from build123d import *

# Parameters (mm, degrees)
SKETCH1_W               = 1019.556
SKETCH1_H               = 756.92
BOSS_EXTRUDE1_DEPTH     = 800
CUT_EXTRUDE1_DEPTH      = 1351.083852483
CUT_EXTRUDE2_DEPTH      = 1022.325404014
CUT_EXTRUDE2_DEPTH_BACK = 1022.325404014


with BuildPart() as part:
    # Sketch1 → Boss-Extrude1 (new body)
    with BuildSketch(Plane.XY):
        Rectangle(SKETCH1_W, SKETCH1_H)
    extrude(amount=BOSS_EXTRUDE1_DEPTH)

    # Sketch2 → Cut-Extrude1 (cut, through all)
    with BuildSketch(Plane(origin=(509.778, 0, 0), x_dir=(0, 0, -1), z_dir=(1, 0, 0))):
        Polygon((2016.625671317, 1289.001404615), (0, 378.46), (-838.195987242, 0), (0, -378.46), (2016.625671317, -1289.001404615), (-2408.694542061, -1289.001404615), (-2408.694542061, 1289.001404615), align=None)
    extrude(amount=-CUT_EXTRUDE1_DEPTH, mode=Mode.SUBTRACT)

    # Sketch4 → Cut-Extrude2 (cut, two sides: drawn at the far end of the back side and taken through both)
    with BuildSketch(Plane(origin=(0, 0, 0), x_dir=(1, 0, 0), z_dir=(0, 1, 0)).offset(-CUT_EXTRUDE2_DEPTH_BACK)):
        Polygon((-1849.85876024, 2230.26891396), (-509.778, 0), (0, -848.413065954), (509.778, 0), (1849.85876024, 2230.26891396), (1849.85876024, -2973.543485633), (-1849.85876024, -2973.543485633), align=None)
    extrude(amount=CUT_EXTRUDE2_DEPTH + CUT_EXTRUDE2_DEPTH_BACK, mode=Mode.SUBTRACT)


solid = part.part
The listing builds one solid part. Answer for the finished solid, in the listing's coordinates (mm). Coordinates: 2 decimals unless noted, no trailing zeros. Write each loop counter-clockwise with the first axis right and the second up, starting at its lowest first coordinate (ties: lowest second). Pieces come first, ordered by that corner, then holes. Notation, with made-up numbers: M 32.5,28.25 L 53.5,28.25 A35 ccw 53.5,64.25 Z; hole C -26.5,59.25 d9. An arc over 180 degrees is marked long. Use one line per item in the form item = value.
Item 1: The mould has two halves that part along X. Classify faces 1 (the face through (-319.48, -5.3, 316.71)), 2 (the face through (7.137, -240.516, 305.511)), 3 (the face through (326.21, -5.3, 305.51)): released by +X, released by -X, zero draft, split by the parting line, or undercut.
Model answer:
face_1 = released by -X
face_2 = zero draft
face_3 = released by +X
Item 2: Given P1, Ø1, axis at x = -27, z = 332.5, coming from the +Y side; P2, Ø10, axis at x = -138, y = -216.5, coming from the +Z side; P3, Ø1, axis at y = 187, z = 390.5, coming from the +X side, each flat-ended and moving along its own axis, determine where each tip first touches the part or whether it passes through.
Model answer:
P1 = 228.56
P2 = 369.78
P3 = 275.44
Item 3: Find section A-A, the plane z = 231. Give the vertices of the cut face in (x, y).
Model answer:
outline = M -370.98,-274.16 L 370.98,-274.16 L 370.98,274.16 L -370.98,274.16 Z
Item 4: Find section B-B, the plane x = 348.5. Give the vertices of the cut face in (y, z).
Model answer:
outline = M -378.46,0 L 378.46,0 L 257.27,268.41 L -257.27,268.41 Z
Item 5: Find the intervals of material crossed by probe 1 along Y at (x, z) = (-99.5, 441.5); probe 2 along X at (y, z) = (89, 462); probe 3 along X at (y, z) = (-257.5, 264), in increasing order.
Model answer:
probe_1 = -179.12 to 179.12
probe_2 = -232.18 to 232.18
probe_3 = -351.15 to 351.15
